```python
from build123d import *

# Parameters (mm, degrees)
SCHIZZO1_R                    = 16
ESTRUSIONE_ESTRUSIONE2_DEPTH  = 3
SCHIZZO2_R                    = 8
ESTRUSIONE_ESTRUSIONE3_DEPTH  = 10
SCHIZZO3_R                    = 4
SCHIZZO3_R_2                  = 2
TAGLIO_ESTRUSIONE1_DEPTH      = 1
TAGLIO_ESTRUSIONE1_DEPTH_BACK = 14
SCHIZZO4_R                    = 1.5
TAGLIO_ESTRUSIONE2_DEPTH      = 17
TAGLIO_ESTRUSIONE2_DEPTH_BACK = 17


with BuildPart() as part:
    # Schizzo1 → Estrusione-Estrusione2 (new body)
    with BuildSketch(Plane.XY):
        Circle(SCHIZZO1_R)
    extrude(amount=ESTRUSIONE_ESTRUSIONE2_DEPTH)

    # Schizzo2 → Estrusione-Estrusione3 (add)
    with BuildSketch(Plane.XY.offset(3)):
        Circle(SCHIZZO2_R)
    extrude(amount=ESTRUSIONE_ESTRUSIONE3_DEPTH)

    # Schizzo3 → Taglio-Estrusione1 (cut, two sides)
    with BuildSketch(Plane.XY.offset(13)) as taglio_estrusione1_sk:
        Circle(SCHIZZO3_R)
        with Locations((12, 0)):
            Circle(SCHIZZO3_R_2)
        with Locations((0, 12)):
            Circle(SCHIZZO3_R_2)
        with Locations((-12, 0)):
            Circle(SCHIZZO3_R_2)
        with Locations((0, -12)):
            Circle(SCHIZZO3_R_2)
    extrude(amount=TAGLIO_ESTRUSIONE1_DEPTH, mode=Mode.SUBTRACT)
    extrude(taglio_estrusione1_sk.sketch, amount=-TAGLIO_ESTRUSIONE1_DEPTH_BACK, mode=Mode.SUBTRACT)

    # Schizzo4 → Taglio-Estrusione2 (cut, two sides)
    with BuildSketch(Plane(origin=(0, 0, 0), x_dir=(1, 0, 0), z_dir=(0, 1, 0))) as taglio_estrusione2_sk:
        with Locations((0, -8)):
            Circle(SCHIZZO4_R)
    extrude(amount=TAGLIO_ESTRUSIONE2_DEPTH, mode=Mode.SUBTRACT)
    extrude(taglio_estrusione2_sk.sketch, amount=-TAGLIO_ESTRUSIONE2_DEPTH_BACK, mode=Mode.SUBTRACT)


solid = part.part
```
Model file for the job. Use its own axes, mm. A direction names the side the tool comes from. Round coordinates to 2 decimals unless told otherwise and drop trailing zeros. Write each loop counter-clockwise with the first axis right and the second up, starting at its lowest first coordinate (ties: lowest second). Pieces come first, ordered by that corner, then holes. Notation, with made-up numbers: (-39.75, 71) -> (12.25, 71) arc R8 ccw to (12.25, 84) -> close; hole circle Ø2 at (-11, 28). An arc over 180 degrees is marked (long way). Answer as CSV lines item,"result".
1. Pin check, flat tips, straight feed: pin 1 Ø3 at (x, z) = (-5, 11) entering from +Y; pin 2 Ø3.5 at (x, z) = (0, 8) entering from -Y; pin 3 Ø5 at (x, z) = (6, 3) entering from -Y; pin 4 Ø3.5 at (x, y) = (-12, 0) entering from -Z. Stop position of each tip, or through.
Resolved:
pin 1,"y = 7.19"
pin 2,"y = -8"
pin 3,"y = -15.61"
pin 4,"through"
2. Slice it at D-D, the plane x = 12. List the corners of the cut face in (y, z), plus the area to 3 significant figures.
Resolved:
outline,"(-10.58, 0) -> (-2, 0) -> (-2, 3) -> (-10.58, 3) -> close; (2, 0) -> (10.58, 0) -> (10.58, 3) -> (2, 3) -> close"
area,"51.5 mm²"
3. Slice it at C-C, the plane z = 8.75. List the corners of the cut face in (x, y).
Resolved:
outline,"(-1.3, -7.89) -> (-1.3, -3.78) arc R4 cw to (-1.3, 3.78) -> (-1.3, 7.89) arc R8 ccw to start; (1.3, -7.89) arc R8 ccw to (1.3, 7.89) -> (1.3, 3.78) arc R4 cw to (1.3, -3.78) -> close"
4. Drill centre lines: line 1 (Y direction, x = 0, z = 9.75); line 2 (Z direction, x = 0, y = 4.8); line 3 (Z direction, x = 4, y = -11.5). Where is each one in solid material? Low to high.
Resolved:
line 1,"-8 to -4, 4 to 8"
line 2,"0 to 6.5, 9.5 to 13"
line 3,"0 to 3"
5. Mould opens along Y. For faces 3 (the face through (-1.5, -5.83, 7.93)), 4 (the face through (0, -10, 2)), 5 (the face through (3.695, -1.532, 6.591)), 6 (the face through (-1.73, -7.81, 7.93)) say: +Y half, -Y half, draft (parallel to the pull), parting line (faces both ways), or undercut.
Resolved:
face 3,"draft"
face 4,"undercut"
face 5,"undercut"
face 6,"parting line"
6. Slice it at B-B, the plane y = -3. List the corners of the cut face in (x, z), plus the area to 3 significant figures.
Resolved:
outline,"(-15.72, 0) -> (-2.65, 0) -> (-2.65, 13) -> (-7.42, 13) -> (-7.42, 3) -> (-15.72, 3) -> close; (2.65, 0) -> (15.72, 0) -> (15.72, 3) -> (7.42, 3) -> (7.42, 13) -> (2.65, 13) -> close"
area,"174 mm²"
7. Slice it at A-A, the plane x = 0. List the corners of the cut face in (y, z), plus the area to 3 significant figures.
Resolved:
outline,"(-16, 0) -> (-14, 0) -> (-14, 3) -> (-16, 3) -> close; (-10, 0) -> (-4, 0) -> (-4, 6.5) -> (-8, 6.5) -> (-8, 3) -> (-10, 3) -> close; (-8, 9.5) -> (-4, 9.5) -> (-4, 13) -> (-8, 13) -> close; (4, 0) -> (10, 0) -> (10, 3) -> (8, 3) -> (8, 6.5) -> (4, 6.5) -> close; (4, 9.5) -> (8, 9.5) -> (8, 13) -> (4, 13) -> close; (14, 0) -> (16, 0) -> (16, 3) -> (14, 3) -> close"
area,"104 mm²"
8. Tool access for faces 1 (the face through (3, -3, 0)), 2 (the face through (-3.8, 7.3, 3)): list every direction of +Z, -Z, +X, -X, +Y, -Y with a clear straight run to the whole face (end or side of a thin tool).
Resolved:
face 1,"-Z, +X, -X, +Y, -Y"
face 2,"+Z"
